Design review of the part built by this model. Coordinates are the model's own, in mm. A direction names the side the tool comes from. Coordinates: 2 decimals unless noted, no trailing zeros. Order: outer loops, then holes, each group sorted by start corner. A loop starts at its lowest first (then second) coordinate and runs counter-clockwise, first axis right, second up. Notation, with made-up numbers: (64.25, -25.75) -> (79.25, -25.75) arc R23 ccw to (79.25, 0.25) -> close; hole circle Ø4 at (-6, 35.25). An arc over 180 degrees is marked (long way). Use a Markdown table: item, result. Add a question column.
Q1. Add section D-D (x = 30.5). State the section outline as (y, z) points, then the cut area to 4 significant figures.
Q2. Machinability: for faces 4 (the face through (0, 3, 11)), 5 (the face through (3.912, 5.148, 20.472)), 6 (the face through (6, 3, 16.5)), which of the approach directions +Z, -Z, +X, -X, +Y, -Y give a long, thin tool a straight path to every point of the face, cutting with its end or side? Answer none if there is none.
Q3. Insertion check: pin 1 (1.9 mm diameter, centred on y = 3, z = 6.5, fed in from +X). The pin has a flat end and moves straight along its axis. Give the tip position at first contact, or say it passes through.
Q4. Add section C-C (x = 5). State the section outline as (y, z) points, then the cut area to 3 significant figures.
Q5. Add section A-A (z = 19.5). State the section outline as (x, y) points, then the cut area to 3 significant figures.
Q6. The part is to be moulded in two halves that separate along Z. For faces 1 (the face through (4, 3, 9)), 2 (the face through (4.1, 1, 22.5)), 3 (the face through (8, 3, 19)), say which applies: pulls with the +Z half, pulls with the -Z half, needs draft (parallel to the pull), parting line crosses it, or undercut.
Q7. Wall thickness on probe 1 along Y at (x, z) = (4, 19.85); probe 2 along X at (y, z) = (3.15, 20.8); probe 3 along Z at (x, y) = (49, 4.25): over which ranges is each line inside the solid? List them lowest first.
Q8. Add section B-B (y = 0.5). State the section outline as (x, z) points.
Autodesk Fusion 360 part; units mm, degrees
sketch "Sketch1" plane through (0, 0, 0) normal (0, 0, 1) x (1, 0, 0)
  line L0 (0, 0) -> (55, 0)
  line L1 (55, 0) -> (55, 6.3)
  line L2 (55, 6.3) -> (0, 6.3)
  line L3 (0, 6.3) -> (0, 0)
  dimension "d1" = 55
  dimension "d2" = 6.3
extrude "Extrude1" add sketch "Sketch1" along normal blind 2.5 makes body 1
sketch "Sketch2" plane through (0, 0, 2.5) normal (0, 0, 1) x (-1, 0, 0)
  line L0 (0, -6.3) -> (0, 0)
  line L1 (0, 0) -> (-55, 0)
  line L2 (-55, 0) -> (-55, -6.3)
  line L3 (-55, -6.3) -> (0, -6.3)
  line L4 (0, 0) -> (-4, 0)
  line L5 (-4, 0) -> (-4, -6.3)
  line L6 (-4, -6.3) -> (0, -6.3)
  line L7 (0, -6.3) -> (0, 0)
  dimension "d5" = 4
extrude "Extrude2" add sketch "Sketch2" along normal blind 14 contours L0 L1 L3 L4 L5 L6 L7 bodies 1
sketch "Sketch3" plane through (0, 0, 16.5) normal (0, 0, 1) x (-1, 0, 0)
  line L0 (0, -6.3) -> (0, 0)
  line L1 (0, 0) -> (-4, 0)
  line L2 (-4, 0) -> (-4, -6.3)
  line L3 (-4, -6.3) -> (0, -6.3)
  line L4 (0, 0) -> (-8, 0)
  line L5 (-8, 0) -> (-8, -6.3)
  line L6 (-8, -6.3) -> (0, -6.3)
  line L7 (0, -6.3) -> (0, 0)
  dimension "d8" = 8
  dimension "d9" = 6.3
extrude "Extrude3" add sketch "Sketch3" along normal blind 6 bodies 1
hole "Hole1" at (4, 3.15, 22.5) direction (0, 0, -1) diameter 4 depth 4 tip angle 180 bodies 1
copy_body "Body->Comp1" bodies 1 removing the originals makes body 2 in component "Hook v2 (1)"
component "Hook v2 (1)" placed x (1, 0, 0) y (0, 1, 0) z (0, 0, 1) at (0, 0, 0)
Established:
| question | item | result |
|---|---|---|
| 1 | outline | (0, 0) -> (6.3, 0) -> (6.3, 2.5) -> (0, 2.5) -> close |
| 1 | area | 15.75 mm^2 |
| 2 | face 4 | +Z, -Z, -X, +Y, -Y |
| 2 | face 5 | +Z |
| 2 | face 6 | +X, +Y, -Y |
| 3 | pin 1 | x = 4 |
| 4 | outline | (0, 0) -> (6.3, 0) -> (6.3, 2.5) -> (0, 2.5) -> close; (0, 16.5) -> (6.3, 16.5) -> (6.3, 22.5) -> (4.88, 22.5) -> (4.88, 18.5) -> (1.42, 18.5) -> (1.42, 22.5) -> (0, 22.5) -> close |
| 4 | area | 39.7 mm^2 |
| 5 | outline | (0, 0) -> (8, 0) -> (8, 6.3) -> (0, 6.3) -> close; hole circle Ø4 at (4, 3.15) |
| 5 | area | 37.8 mm^2 |
| 6 | face 1 | undercut |
| 6 | face 2 | pulls with the +Z half |
| 6 | face 3 | needs draft |
| 7 | probe 1 | 0 to 1.15, 5.15 to 6.3 |
| 7 | probe 2 | 0 to 2, 6 to 8 |
| 7 | probe 3 | 0 to 2.5 |
| 8 | outline | (0, 0) -> (55, 0) -> (55, 2.5) -> (4, 2.5) -> (4, 16.5) -> (8, 16.5) -> (8, 22.5) -> (0, 22.5) -> close |
